Autodesk Fusion 360 part; units mm, degrees
sketch "Sketch1" plane through (0, 0, 0) normal (0, 0, 1) x (1, 0, 0)
  circle A0 centre (0, 0) radius 100
  dimension "d1" = 200
extrude "Extrude1" add sketch "Sketch1" along normal blind 100
sketch "Sketch2" plane through (0, 0, 0) normal (0, 0, -1) x (1, 0, 0)
  circle A0 centre (0, 0) radius 100
  circle A1 centre (0, 0) radius 10
  dimension "d4" = 20
extrude "Extrude2" cut sketch "Sketch2" against normal blind 25 contours A1
sketch "Sketch3" plane through (0, 0, 0) normal (0, 1, 0) x (1, 0, 0)
  circle A0 centre (0, -170) radius 35
  line L0 (-62.5, -170) -> (-62.5, -100)
  line L1 (-62.5, -100) -> (62.5, -100)
  line L2 (62.5, -170) -> (62.5, -100)
  arc A1 (-62.5, -170) -> (62.5, -170) centre (0, -170) ccw
  dimension "d7" = 70
  dimension "d8" = 125
  dimension "d9" = 125
extrude "Extrude3" add sketch "Sketch3" along normal mid plane 50
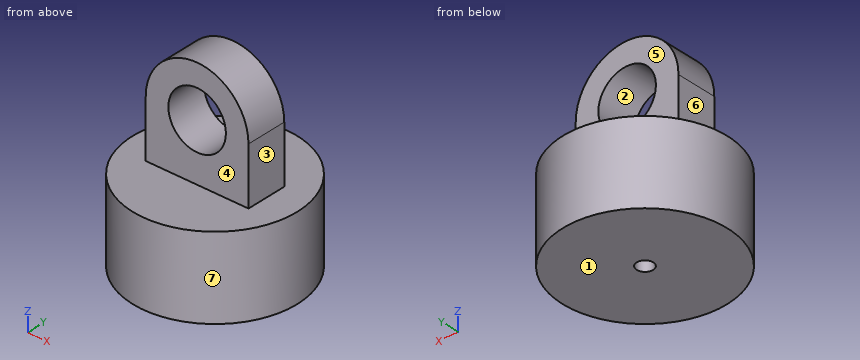
The listing builds one solid part. Answer for the finished solid, in the listing's coordinates (mm). Face numbers are marked on the shaded views. A direction names the side the tool comes from. Give positions to 0.01 mm unless a question says otherwise; leave off trailing zeros. Order: outer loops, then holes, each group sorted by start corner. A loop starts at its lowest first (then second) coordinate and runs counter-clockwise, first axis right, second up.
1) Given P1, Ø4, axis at y = -39.5, z = 92, coming from the -X side; P2, Ø12, axis at x = 0, y = 0, coming from the +Z side; P3, Ø10, axis at y = 49, z = 98, coming from the +X side; P4, Ø16, axis at x = 4, y = 3, coming from the -Z side, each flat-ended and moving along its own axis, determine where each tip first touches the part or whether it passes through.
Reported:
P1: stops at x = -92.7
P2: stops at z = 232.5
P3: stops at x = 89.8
P4: stops at z = 0
2) Consider line 1 along Z through (x, y) = (0, -6); line 2 along X through (y, z) = (4, 170); line 3 along Y through (x, z) = (0, 7). Determine where each line is inside the solid, lowest interval first.
Reported:
line 1: z = 25 to 135, 205 to 232.5
line 2: x = -62.5 to -35, 35 to 62.5
line 3: y = -100 to -10, 10 to 100
3) Determine the mould class of the marked faces 1, 2 and 3 for opening direction X: pulls with the +X half, pulls with the -X half, needs draft (parallel to the pull), parting line crosses it, or undercut.
Reported:
face 1: needs draft
face 2: undercut
face 3: pulls with the +X half
4) Find section B-B on z = 173. Write down the section's boundary in (x, y), then the cut area to 3 significant figures.
Reported:
outline: (-62.43, -25) - (-34.87, -25) - (-34.87, 25) - (-62.43, 25) - close; (34.87, -25) - (62.43, -25) - (62.43, 25) - (34.87, 25) - close
area: 2,760 mm2
5) Find section A-A on x = 0. Write down the section's boundary in (y, z), then the cut area to 3 significant figures.
Reported:
outline: (-100, 0) - (-10, 0) - (-10, 25) - (10, 25) - (10, 0) - (100, 0) - (100, 100) - (25, 100) - (25, 135) - (-25, 135) - (-25, 100) - (-100, 100) - close; (-25, 205) - (25, 205) - (25, 232.5) - (-25, 232.5) - close
area: 22,600 mm2
6) Find section C-C on y = 0. Write down the section's boundary in (x, z), then the cut area to 3 significant figures.
Reported:
outline: (-100, 0) - (-10, 0) - (-10, 25) - (10, 25) - (10, 0) - (100, 0) - (100, 100) - (62.5, 100) - (62.5, 170) arc R62.5 ccw to (-62.5, 170) - (-62.5, 100) - (-100, 100) - close; hole circle Ø70 at (0, 170)
area: 30,500 mm2
7) For the marked faces 4, 5, 6 and 7, determine the directions among +Z, -Z, +X, -X, +Y, -Y from which every point of the face is accessible in a straight line to the end or side of a thin tool.
Reported:
face 4: +Z, +X, -X, -Y
face 5: +Z, +X, -X, +Y
face 6: +Z, -X, +Y, -Y
face 7: +Z, -Z
8) Find section D-D on x = 21.5. Write down the section's boundary in (y, z), then the cut area to 3 significant figures.
Reported:
outline: (-97.66, 0) - (97.66, 0) - (97.66, 100) - (25, 100) - (25, 142.38) - (-25, 142.38) - (-25, 100) - (-97.66, 100) - close; (-25, 197.62) - (25, 197.62) - (25, 228.69) - (-25, 228.69) - close
area: 23,200 mm2
